Build history of the part. All positions in model axes, mm. Face numbers are marked on the shaded views. A direction names the side the tool comes from. Coordinates: 2 decimals unless noted, no trailing zeros. Loops run counter-clockwise (first coordinate to the right, second up) from the corner with the lowest first, then second, coordinate; pieces in that order, holes last.
(1) Slice it at A-A (x = 8). Give the cut face in (y, z).
(2) Two-plate mould, pull along Y, no slides. Class the marked faces 6, 7 and 8: pulls with the +Y half, pulls with the -Y half, needs draft (parallel to the pull), parting line crosses it, or undercut.
(3) Tool access for the marked faces 1, 2, 3, 4 and 5: list every direction of +Z, -Z, +X, -X, +Y, -Y with a clear straight run to the whole face (end or side of a thin tool).
(4) Slice it at B-B (y = 14). Give the cut face in (x, z), and give its area (3 significant figures).
(5) Flat gauge pins, fed straight in: P1, Ø11, axis at x = -30, y = -6.5, coming from the +Z side; P2, Ø2, axis at y = 2.5, z = 47.5, coming from the +X side; P3, Ø25, axis at x = -12, y = -1.5, coming from the -Z side; P4, Ø8, axis at y = -18.5, z = 36.5, coming from the -X side. Where does each tip first touch, or does it go through?
(6) Wall check: L1, parallel to Y at x = -30.5, z = 70; L2, parallel to X at y = 24, z = 95.5. Give the ranges that are in metal, low to high.
from build123d import *

# Parameters (mm, degrees)
SKETCH_1_W          = 70
SKETCH_1_H          = 70
EXTRUDE_1_DEPTH     = 10
SKETCH_2_R          = 17.5
SKETCH_2_W          = 15.660204931
SKETCH_2_H          = 43.06556356
EXTRUDE_2_DEPTH     = 35
SKETCH_2_2_R        = 17.5
SKETCH_2_2_W        = 15.660204931
SKETCH_2_2_H        = 43.06556356
CUT_EXTRUDE_1_DEPTH = 25
SKETCH_3_R          = 17.5
SKETCH_3_W          = 15.660204931
SKETCH_3_H          = 43.06556356
EXTRUDE_3_DEPTH     = 35
SKETCH_3_3_R        = 17.5
SKETCH_3_3_W        = 15.660204931
SKETCH_3_3_H        = 43.06556356
CUT_EXTRUDE_2_DEPTH = 25


with BuildPart() as part:
    # 草圖1 → 填料-伸長1 (new body)
    with BuildSketch(Plane.XY):
        Rectangle(SKETCH_1_W, SKETCH_1_H)
    extrude(amount=EXTRUDE_1_DEPTH)

    # 草圖2 → 填料-伸長2 (add, symmetric)
    with BuildSketch(Plane(origin=(0, 0, 0), x_dir=(0, 0, -1), z_dir=(1, 0, 0))):
        with BuildLine():
            Line((-10, 35), (-70, 35))
            ThreePointArc((-70, 35), (-105.476695364, -0.476695364), (-70, -35.953390728))
            Line((-70, -35.953390728), (-10, -35))
            Line((-10, -35), (-10, 35))
        make_face()
        with Locations((-70, -0.476695364)):
            Circle(SKETCH_2_R, mode=Mode.SUBTRACT)
        with Locations((-34.843422831, -1.110145808)):
            Rectangle(SKETCH_2_W, SKETCH_2_H, mode=Mode.SUBTRACT)
    extrude(amount=EXTRUDE_2_DEPTH, both=True)

    # 草圖2<2> → 除料-伸長1 (cut, symmetric)
    with BuildSketch(Plane(origin=(0, 0, 0), x_dir=(0, 0, -1), z_dir=(1, 0, 0))):
        with BuildLine():
            Line((-10, 35), (-70, 35))
            ThreePointArc((-70, 35), (-105.476695364, -0.476695364), (-70, -35.953390728))
            Line((-70, -35.953390728), (-10, -35))
            Line((-10, -35), (-10, 35))
        make_face()
        with Locations((-70, -0.476695364)):
            Circle(SKETCH_2_2_R, mode=Mode.SUBTRACT)
        with Locations((-34.843422831, -1.110145808)):
            Rectangle(SKETCH_2_2_W, SKETCH_2_2_H, mode=Mode.SUBTRACT)
    extrude(amount=CUT_EXTRUDE_1_DEPTH, both=True, mode=Mode.SUBTRACT)

    # 草圖3 → 填料-伸長3 (add, symmetric)
    with BuildSketch(Plane(origin=(0, 0, 10), x_dir=(0, 0, 1), z_dir=(0, -1, 0))):
        with BuildLine():
            Line((-10, 35), (-70, 35))
            ThreePointArc((-70, 35), (-105.476695364, -0.476695364), (-70, -35.953390728))
            Line((-70, -35.953390728), (-10, -35))
            Line((-10, -35), (-10, 35))
        make_face()
        with Locations((-70, -0.476695364)):
            Circle(SKETCH_3_R, mode=Mode.SUBTRACT)
        with Locations((-34.843422831, -1.110145808)):
            Rectangle(SKETCH_3_W, SKETCH_3_H, mode=Mode.SUBTRACT)
    extrude(amount=EXTRUDE_3_DEPTH, both=True)

    # 草圖3<3> → 除料-伸長2 (cut, symmetric)
    with BuildSketch(Plane(origin=(0, 0, 10), x_dir=(0, 0, 1), z_dir=(0, -1, 0))):
        with BuildLine():
            Line((-10, 35), (-70, 35))
            ThreePointArc((-70, 35), (-105.476695364, -0.476695364), (-70, -35.953390728))
            Line((-70, -35.953390728), (-10, -35))
            Line((-10, -35), (-10, 35))
        make_face()
        with Locations((-70, -0.476695364)):
            Circle(SKETCH_3_3_R, mode=Mode.SUBTRACT)
        with Locations((-34.843422831, -1.110145808)):
            Rectangle(SKETCH_3_3_W, SKETCH_3_3_H, mode=Mode.SUBTRACT)
    extrude(amount=CUT_EXTRUDE_2_DEPTH, both=True, mode=Mode.SUBTRACT)


solid = part.part
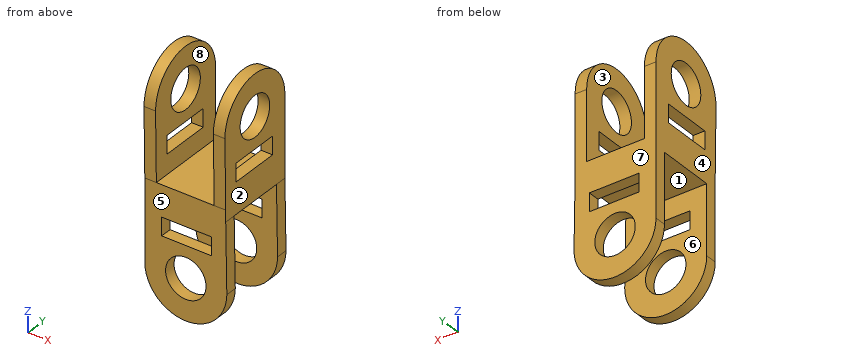
Response values:
1. outline: (-35, -94.67) - (-25, -94.67) - (-25, -75.8) - (-35, -75.8) - close; (-35, -44.2) - (-25, -44.2) - (-25, -32.67) - (-35, -32.67) - close; (-35, -17.01) - (-25, -17.01) - (-25, 0) - (25, 0) - (25, -17.01) - (35, -17.01) - (35, 10) - (-35, 10) - close; (25, -94.67) - (35, -94.67) - (35, -75.8) - (25, -75.8) - close; (25, -44.2) - (35, -44.2) - (35, -32.67) - (25, -32.67) - close
2. face 6: undercut
2. face 7: pulls with the +Y half
2. face 8: needs draft
3. face 1: -Z, +X, -X
3. face 2: +Z, +X, +Y, -Y
3. face 3: +Z, +Y, -Y
3. face 4: +Z, -Z, -X, +Y, -Y
3. face 5: -Z, +X, -X, -Y
4. outline: (-35, 0) - (35, 0) - (35, 27.01) - (25, 27.01) - (25, 10) - (-25, 10) - (-25, 27.01) - (-35, 27.01) - close; (-35, 42.67) - (-25, 42.67) - (-25, 60.17) - (-35, 60.17) - close; (-35, 79.83) - (-25, 79.83) - (-25, 102.39) - (-35, 102.39) - close; (25, 42.67) - (35, 42.67) - (35, 60.17) - (25, 60.17) - close; (25, 79.83) - (35, 79.83) - (35, 102.39) - (25, 102.39) - close
4. area: 1,840 mm2
5. P1: stops at z = 105.47
5. P2: stops at x = 35
5. P3: stops at z = 0
5. P4: passes through
6. L1: y = -35.95 to -17.98, 17.02 to 35
6. L2: x = -35 to -25, 25 to 35
